Verification items for the finished model (mm, model axes). A direction names the side the tool comes from. Coordinates: 2 decimals unless noted, no trailing zeros. Write item = value, one per line.
```python
from build123d import *

# Parameters (mm, degrees)
SKETCH7_R           = 14
SKETCH7_R_2         = 13
BOSS_EXTRUDE2_DEPTH = 4
BOSS_EXTRUDE6_START = 3.5
SKETCH7_3_R         = 14
BOSS_EXTRUDE6_DEPTH = 0.5
THREAD3_PITCH       = 1


with BuildPart() as part:
    # Sketch7 → Boss-Extrude2 (new body)
    with BuildSketch(Plane(origin=(0, 0, 0), x_dir=(1, 0, 0), z_dir=(0, 1, 0))):
        with Locations(Location((40, 0, 0), (0, 0, 270))):
            Circle(SKETCH7_R)
        with Locations(Location((40, 0, 0), (0, 0, 270))):
            Circle(SKETCH7_R_2, mode=Mode.SUBTRACT)
    extrude(amount=BOSS_EXTRUDE2_DEPTH)

    # Sketch7<3> → Boss-Extrude6 (add)
    with BuildSketch(Plane(origin=(0, 0, 0), x_dir=(1, 0, 0), z_dir=(0, 1, 0)).offset(BOSS_EXTRUDE6_START)):
        with Locations(Location((40, 0, 0), (0, 0, 270))):
            Circle(SKETCH7_3_R)
    extrude(amount=BOSS_EXTRUDE6_DEPTH)

    # Thread3: arcs per turn and ends read off the stored shape
    # Thread3: the profile of Thread Profile3 profile screwed along a right-hand helix through 4 turns, 8 arcs to a turn; built about Z, then put on its axis
    thread3_z = Axis((0, 0, 0), (0, 0, 1))
    thread3_corners = [(12.9997, 0, -0.000173205), (13.541265875, 0, 0.312499999), (13.541265875, 0, 0.437499999), (12.9997, 0, 0.750173202)]
    with BuildLine(mode=Mode.PRIVATE) as thread3_profile:
        Line(thread3_corners[0], thread3_corners[1])
        Line(thread3_corners[1], thread3_corners[2])
        Line(thread3_corners[2], thread3_corners[3])
        Line(thread3_corners[3], thread3_corners[0])
    thread3_cap = Face(thread3_profile.wire())
    thread3_turn_angles = [0, 22.5, 45, 67.5, 90, 112.5, 135, 157.5, 180, 202.5, 225, 247.5, 270, 292.5, 315, 337.5, 360]
    thread3_turn_weights = [1, 0.9238795325112867, 1, 0.9238795325112867, 1, 0.9238795325112867, 1, 0.9238795325112867, 1, 0.9238795325112867, 1, 0.9238795325112867, 1, 0.9238795325112867, 1, 0.9238795325112867, 1]
    thread3_turn_rails = [Edge.make_bspline([Vector(p[0], p[1], 0).rotate(thread3_z, thread3_turn_angles[k]) / thread3_turn_weights[k] + Vector(0, 0, p[2] + THREAD3_PITCH * thread3_turn_angles[k] / 360) for k in range(17)], [0, 0, 0, 1, 1, 2, 2, 3, 3, 4, 4, 5, 5, 6, 6, 7, 7, 8, 8, 8], 2, thread3_turn_weights) for p in thread3_corners]
    thread3_turn_sides = [Face.make_surface_from_curves(thread3_turn_rails[p[0]], thread3_turn_rails[p[1]]) for p in [(0, 1), (1, 2), (2, 3), (3, 0)]]
    thread3 = Plane(origin=(40, 3.5, 0), x_dir=(-1, 0, 0), z_dir=(0, -1, 0)) * Solid(Shell([*[p.moved(Location((0, 0, THREAD3_PITCH * i))) for i in range(4) for p in thread3_turn_sides], thread3_cap, thread3_cap.rotate(thread3_z, 1440).moved(Location((0, 0, THREAD3_PITCH * 1440 / 360)))]))
    add(thread3, mode=Mode.SUBTRACT)


solid = part.part
```
Item 1: Tool access check on faces 1 (the flat face through (40, 3.5, 0)), 2 (the flat face through (40, 4, 0)). Record the directions out of +Z, -Z, +X, -X, +Y, -Y that give a thin tool (end or side, any length) a straight path to the whole face; none if there is none.
Report:
face_1 = -Y
face_2 = +Z, -Z, +X, -X, +Y
Item 2: Scan lines: L1, parallel to Y at x = 49, z = 6.5; L2, parallel to X at y = 1, z = -3; L3, parallel to Z at x = 42, y = 1.95. Record each from-to range of solid material in increasing order. Write a range as from..to.
Report:
L1 = 3.5..4
L2 = 26.33..26.84, 52.71..53.67
L3 = -13.86..-13.33, 12.85..13.86
Item 3: Gauge pin test, flat ends, axial feed: pin 1 (0.6 mm diameter, centred on x = 27, y = 3, fed in from -Z); pin 2 (5 mm diameter, centred on x = 44.5, z = 7.5, fed in from -Y); pin 3 (2 mm diameter, centred on y = 1, z = 8.5, fed in from +X); pin 4 (12 mm diameter, centred on x = 40, z = 9.5, fed in from -Y). Record the tip position at first contact, or that the pin passes through.
Report:
pin_1 = -5.89
pin_2 = 3.5
pin_3 = 51.82
pin_4 = 0
